from build123d import *

# Parameters (mm, degrees)
SKETCH2_R           = 25.25
BOSS_EXTRUDE1_DEPTH = 25
SKETCH8_W           = 3.6
SKETCH8_H           = 2.3
CIRPATTERN1_COUNT   = 6


with BuildPart() as part:
    # Sketch2 → Boss-Extrude1 (new body)
    with BuildSketch(Plane.XY):
        Circle(SKETCH2_R)
    extrude(amount=BOSS_EXTRUDE1_DEPTH)

    # Sketch6 → Cut-Revolve2 (revolve, cut)
    with BuildSketch(Plane(origin=(0, 0, 0), x_dir=(0, 0, -1), z_dir=(1, 0, 0)), mode=Mode.PRIVATE) as cut_revolve2_sk:
        Polygon((-25, 0), (-25, 8), (-13.59, 8), (-9.799695483, 1.435), (0, 4.06), (0, 0), align=None)
    revolve(cut_revolve2_sk.sketch.rotate(Axis((0, 0, 0), (0, 0, 1)), 90), axis=Axis((0, 0, 0), (0, 0, 1)), mode=Mode.SUBTRACT)

    # Sketch8 → Cut-Revolve3 (revolve, cut)
    with BuildSketch(Plane(origin=(0, 0, 0), x_dir=(0, 0, -1), z_dir=(1, 0, 0)), mode=Mode.PRIVATE) as cut_revolve3_sk:
        with Locations((-13.2, 24.1)):
            Rectangle(SKETCH8_W, SKETCH8_H)
    revolve(cut_revolve3_sk.sketch.rotate(Axis((0, 0, 25), (0, 0, -1)), 90), axis=Axis((0, 0, 25), (0, 0, -1)), mode=Mode.SUBTRACT)

    # Sketch9 → #8-32 Tapped Hole1 (revolve, cut)
    with BuildSketch(Plane(origin=(0.079165003, 25.249875899, 5), x_dir=(-0.9999950850990496, 0.003135247636910079, 0), z_dir=(0, 0, 1))):
        Polygon((0, 0), (0, 11.037806461), (1.7272, 10), (1.7272, 0), align=None)
    f_8_32_tapped_hole1 = revolve(axis=Axis((0.099073825, 31.599844689, 5), (-0.0031352476369100784, -0.9999950850990494, 0)), mode=Mode.SUBTRACT)

    # CirPattern1: #8-32 Tapped Hole1 ×6 about axis
    cirpattern1_axis = Axis((0, 0, 25), (0, 0, -1))
    for i in range(1, CIRPATTERN1_COUNT):
        add(f_8_32_tapped_hole1.rotate(cirpattern1_axis, i * 360 / CIRPATTERN1_COUNT), mode=Mode.SUBTRACT)


solid = part.part
Can you work these out from the model? Positions are in its coordinate system, mm. A direction names the side the tool comes from. Give positions to 0.01 mm unless a question says otherwise; leave off trailing zeros. Loops run counter-clockwise (first coordinate to the right, second up) from the corner with the lowest first, then second, coordinate; pieces in that order, holes last. Notation, with made-up numbers: (47, -12.5) -> (65, -12.5) arc R16 ccw to (65, -6.5) -> close; hole circle Ø7 at (0, 66). An arc over 180 degrees is marked (long way). Use one line per item in the form item = value.
1) For faces 1 (the face through (-12.605, -6.951, 5.183)), 2 (the face through (0, -5, 0)), 3 (the face through (1.73, 7.81, 19.22)), 4 (the face through (0.536, 2.415, 5.92)), which set-ups out of +Z, -Z, +X, -X, +Y, -Y let a thin tool reach every point of the face, with its end or its side?
Answers:
face_1 = none
face_2 = -Z, +X, -X, +Y, -Y
face_3 = +Z
face_4 = -Z
2) If we section it at C-C (z = 16): Please give me the cut outline in (x, y).
Answers:
outline = circle Ø50.5 at (0, 0); hole circle Ø16 at (0, 0)
3) If we section it at B-B (x = -10.5): Please give me the cut outline in (y, z).
Answers:
outline = (-22.96, 0) -> (22.96, 0) -> (22.96, 11.4) -> (20.41, 11.4) -> (20.41, 15) -> (22.96, 15) -> (22.96, 25) -> (-22.96, 25) -> (-22.96, 15) -> (-20.41, 15) -> (-20.41, 11.4) -> (-22.96, 11.4) -> close
4) If we section it at A-A (y = 0): Please give me the cut outline in (x, z) (3 decimals), plus the area to 3 significant figures.
Answers:
outline = (-25.25, 0) -> (-4.06, 0) -> (-1.435, 9.8) -> (-8, 13.59) -> (-8, 25) -> (-25.25, 25) -> (-25.25, 15) -> (-22.95, 15) -> (-22.95, 11.4) -> (-25.25, 11.4) -> close; (1.435, 9.8) -> (4.06, 0) -> (25.25, 0) -> (25.25, 11.4) -> (22.95, 11.4) -> (22.95, 15) -> (25.25, 15) -> (25.25, 25) -> (8, 25) -> (8, 13.59) -> close
area = 974 mm²
5) I need wall thicknesses on line 1 along Y through (x, z) = (0, 18); line 2 along Y through (x, z) = (-21, 22.5); line 3 along X through (y, z) = (20, 4). Which ranges of each line are inside material? Lowest first, please.
Answers:
line_1 = -25.25 to -8, 8 to 25.25
line_2 = -14.02 to 14.02
line_3 = -15.41 to -1.35, 1.47 to 15.41
6) Will these pins go through, and if not, where does the flat tip stop? pin 1 (10 mm diameter, centred on y = 19, z = 12, fed in from -X); pin 2 (2 mm diameter, centred on x = 19.5, z = 16.5, fed in from +Y); pin 3 (5 mm diameter, centred on x = -17, z = 7, fed in from +Y).
Answers:
pin_1 = -20.99
pin_2 = 17.18
pin_3 = 20.67
7) We'd pull the mould along X, two halves only. Please class faces 5 (the face through (-2.988, -22.755, 13.175)), 6 (the face through (-6, 6, 25)), 7 (the face through (0.438, 20.319, 6.686)): released by +X, released by -X, zero draft, split by the parting line, or undercut.
Answers:
face_5 = split by the parting line
face_6 = zero draft
face_7 = undercut
